The model under review builds one solid part; all positions refer to its coordinate system, in mm. Face numbers are marked on the shaded views. A direction names the side the tool comes from. Round coordinates to 2 decimals unless told otherwise and drop trailing zeros. Order: outer loops, then holes, each group sorted by start corner. A loop starts at its lowest first (then second) coordinate and runs counter-clockwise, first axis right, second up. Notation, with made-up numbers: (-6, 17) -> (39, 17) arc R16 cw to (39, 29) -> close; hole circle Ø5 at (24, -2.75). An arc over 180 degrees is marked (long way). Put each result on its own line as item: value. Start each with the question number.
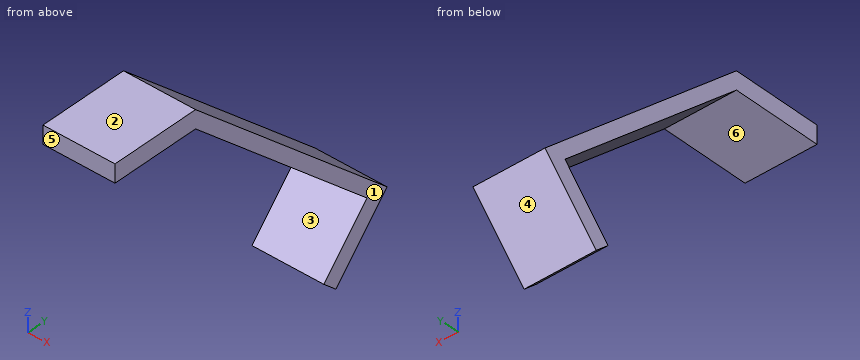
from build123d import *

# Parameters (mm, degrees)
SKETCH1_W           = 12.7
SKETCH1_H           = 63.5
BOSS_EXTRUDE1_DEPTH = 50.8


with BuildPart() as part:
    # Sketch1 → Boss-Extrude1 (new body)
    with BuildSketch(Plane(origin=(0, 0, 0), x_dir=(0, 0, -1), z_dir=(1, 0, 0))):
        Polygon((134.483136253, 198.753875218), (12.7, 63.5), (0, 63.5), (135.967339212, 214.507028537), (180.732852088, 174.199979698), (172.234893387, 164.762040415), align=None)
        with Locations((6.35, 31.75)):
            Rectangle(SKETCH1_W, SKETCH1_H)
    extrude(amount=BOSS_EXTRUDE1_DEPTH)


solid = part.part
Q1. Take a section at B-B on x = 35. Give the boundary of the cut face in (y, z).
Q2. Draft analysis for pull direction Z (two halves, no side actions). For the marked faces 1, 2, 3 and 4, state which applies: +Z half, -Z half, draft (parallel to the pull), parting line (faces both ways), or undercut.
Q3. Take a section at C-C on y = 33. Give the boundary of the cut face in (x, z), and give its area (3 significant figures).
Q4. Wall thickness on probe 1 along Z at (x, y) = (18.5, 11.5); probe 2 along Z at (x, y) = (23, 172); probe 3 along Z at (x, y) = (48, 174.5): over which ranges is each line inside the solid? List them lowest first. Write a range as [from, to].
Q5. For the marked faces 5 and 6, list the 3-axis set-ups (+Z, -Z, +X, -X, +Y, -Y) from which the entire face can be reached by the end or side of a thin tool; tool diameter is ignored.
Q6. Take a section at D-D on z = -68. Give the boundary of the cut face in (x, y).
Q7. Clearance check with flat-ended pins moving along their axes: pin 1 Ø4 at (x, z) = (30, -82.5) entering from +Y; pin 2 Ø1.5 at (x, y) = (44.5, 26) entering from +Z; pin 3 Ø1.5 at (x, z) = (28, -105.5) entering from +Y; pin 4 Ø3 at (x, z) = (41, -86) entering from -Y. State where each tip first meets the part, or that it passes through.
Q8. Take a section at A-A on y = 170. Give the boundary of the cut face in (x, z).
Calculated:
1. outline: (0, -12.7) -> (63.5, -12.7) -> (198.75, -134.48) -> (164.76, -172.23) -> (174.2, -180.73) -> (214.51, -135.97) -> (63.5, 0) -> (0, 0) -> close
2. face 1: draft
2. face 2: +Z half
2. face 3: undercut
2. face 4: -Z half
3. outline: (0, -12.7) -> (50.8, -12.7) -> (50.8, 0) -> (0, 0) -> close
3. area: 645 mm²
4. probe 1: z = [-12.7, 0]
4. probe 2: z = [-178.75, -164.2], [-110.39, -97.69]
4. probe 3: z = [-180.4, -161.42], [-112.64, -99.94]
5. face 5: +Z, -Z, +X, -X, -Y
5. face 6: -Z, +X, -X, -Y
6. outline: (0, 124.92) -> (50.8, 124.92) -> (50.8, 139.02) -> (0, 139.02) -> close
7. pin 1: stops at y = 157.35
7. pin 2: stops at z = 0
7. pin 3: stops at y = 181.5
7. pin 4: stops at y = 143.24
8. outline: (0, -176.95) -> (50.8, -176.95) -> (50.8, -166.42) -> (0, -166.42) -> close; (0, -108.59) -> (50.8, -108.59) -> (50.8, -95.89) -> (0, -95.89) -> close
